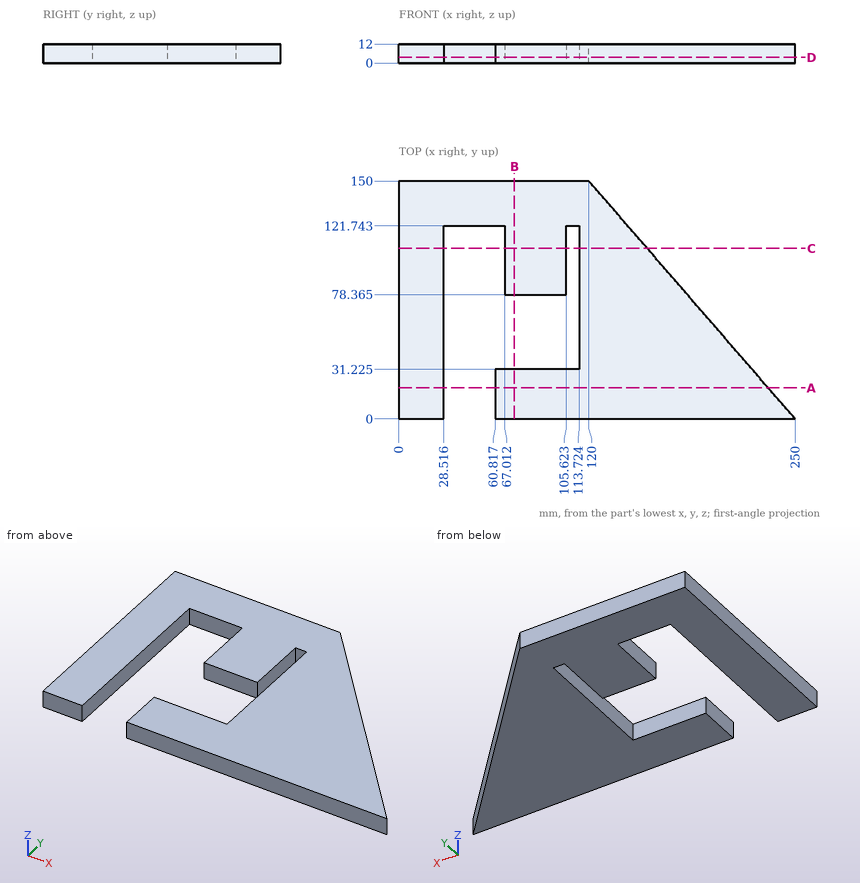
For this review, use the dimensioned drawing (mm, ordinates from the lowest corner) and the shaded views. Round coordinates to 2 decimals unless told otherwise and drop trailing zeros. Loops run counter-clockwise (first coordinate to the right, second up) from the corner with the lowest first, then second, coordinate; pieces in that order, holes last. Notation, with made-up numbers: (15, 75) -> (37, 75) arc R20 ccw to (37, 106) -> close; hole circle Ø6 at (54, 70). An arc over 180 degrees is marked (long way). Write item = value, one per line. Start each with the question number.
Item 1: To check wall thickness, follow L1, parallel to Y at x = 92, z = 2 (1 decimal); L2, parallel to X at y = 92, z = 7.75 (1 decimal); L3, parallel to Y at x = 58, z = 9.75. State the ranges of each line that lie inside material, in increasing order.
Item 2: Take a section at C-C on y = 107.5. Give the boundary of the cut face in (x, z) (1 decimal).
Item 3: Take a section at D-D on z = 3.5. Give the boundary of the cut face in (x, y) (1 decimal), plus the area to 3 significant figures.
Item 4: Take a section at A-A on y = 19.5. Give the boundary of the cut face in (x, z) (1 decimal), plus the area to 3 significant figures.
Item 5: Take a section at B-B on x = 73. Give the boundary of the cut face in (y, z) (1 decimal).
Item 6: Insertion check: pin 1 (6 mm diameter, centred on y = 106.5, z = 5.5, fed in from +X); pin 2 (6 mm diameter, centred on y = 19.5, z = 7.5, fed in from -X); pin 3 (3 mm diameter, centred on y = 18.5, z = 7.5, fed in from +X) (1 decimal); pin 4 (6 mm diameter, centred on y = 66, z = 3.5, fed in from +X). Each pin has a flat end and moves straight along its axis. Give the tip position at first contact, or say it passes through.
Result:
q1.L1 = 0 to 31.2, 78.4 to 150
q1.L2 = 0 to 28.5, 67 to 105.6, 113.7 to 170.3
q1.L3 = 121.74 to 150
q2.outline = (0, 0) -> (28.5, 0) -> (28.5, 12) -> (0, 12) -> close; (67, 0) -> (105.6, 0) -> (105.6, 12) -> (67, 12) -> close; (113.7, 0) -> (156.8, 0) -> (156.8, 12) -> (113.7, 12) -> close
q3.outline = (0, 0) -> (28.5, 0) -> (28.5, 121.7) -> (67, 121.7) -> (67, 78.4) -> (105.6, 78.4) -> (105.6, 121.7) -> (113.7, 121.7) -> (113.7, 31.2) -> (60.8, 31.2) -> (60.8, 0) -> (250, 0) -> (120, 150) -> (0, 150) -> close
q3.area = 20,700 mm²
q4.outline = (0, 0) -> (28.5, 0) -> (28.5, 12) -> (0, 12) -> close; (60.8, 0) -> (233.1, 0) -> (233.1, 12) -> (60.8, 12) -> close
q4.area = 2,410 mm²
q5.outline = (0, 0) -> (31.2, 0) -> (31.2, 12) -> (0, 12) -> close; (78.4, 0) -> (150, 0) -> (150, 12) -> (78.4, 12) -> close
q6.pin_1 = 160.3
q6.pin_2 = 0
q6.pin_3 = 235.3
q6.pin_4 = 195.4
